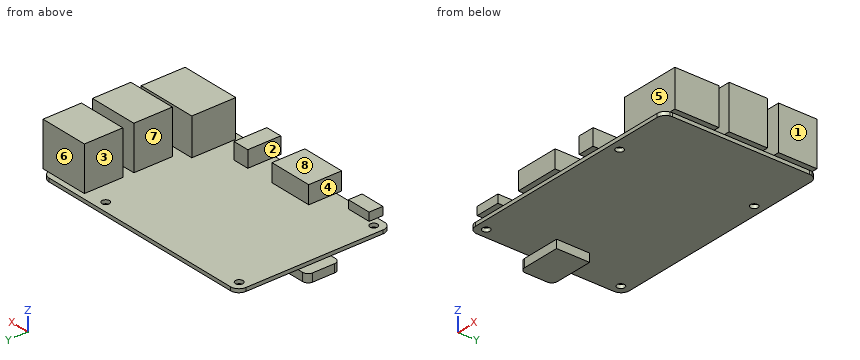
```python
from build123d import *

# Parameters (mm, degrees)
F0_R     = 1.375
F0_W     = 9
F0_H     = 3
F0_W_2   = 16
F0_H_2   = 10
F0_W_3   = 6
F0_H_3   = 14
F1_DEPTH = 1.3
F0_W_4   = 2
F2_DEPTH = 16
F3_DEPTH = 13.5
F0_H_4   = 2
F4_DEPTH = 6
F5_DEPTH = 6.5
F6_DEPTH = 3
F7_W     = 4
F7_H     = 12
F7_W_2   = 12
F8_DEPTH = 3
F9_R     = 2


# Not quite as in the source:
# - a feature names something its author has since deleted; it is built from what else it names


with BuildPart() as f1:
    # F0 (on Top) → F1 (new body)
    with BuildSketch(Plane.XY):
        with BuildLine():
            Line((-28.5, 0), (-3, 0))
            ThreePointArc((-3, 0), (-1.1628826929, 0.6282917549), (-0.0952624903, 2.25))
            Line((-0.0952624903, 2.25), (-20, 2.25))
            Line((-20, 2.25), (-20, 18.25))
            Line((-20, 18.25), (0, 18.25))
            Line((0, 18.25), (0, 22))
            Line((0, 22), (-16, 22))
            Line((-16, 22), (-16, 36))
            Line((-16, 36), (0, 36))
            Line((0, 36), (0, 40))
            Line((0, 40), (-16, 40))
            Line((-16, 40), (-16, 54))
            Line((-16, 54), (-0.1715728753, 54))
            ThreePointArc((-0.1715728753, 54), (-1.2679491924, 55.4494897428), (-3, 56))
            Line((-3, 56), (-82, 56))
            ThreePointArc((-82, 56), (-84.1213203436, 55.1213203436), (-85, 53))
            Line((-85, 53), (-85, 3))
            ThreePointArc((-85, 3), (-84.1213203436, 0.8786796564), (-82, 0))
            Line((-82, 0), (-78.9, 0))
            Line((-78.9, 0), (-78.9, 3))
            Line((-78.9, 3), (-69.9, 3))
            Line((-69.9, 3), (-69.9, 0))
            Line((-69.9, 0), (-61, 0))
            Line((-61, 0), (-61, 10))
            Line((-61, 10), (-45, 10))
            Line((-45, 10), (-45, 0))
            Line((-45, 0), (-34.5, 0))
            Line((-34.5, 0), (-34.5, 10))
            Line((-34.5, 10), (-28.5, 10))
            Line((-28.5, 10), (-28.5, 0))
        make_face()
        with Locations((-81.5, 3.5)):
            Circle(F0_R, mode=Mode.SUBTRACT)
        with Locations((-23.5, 3.5)):
            Circle(F0_R, mode=Mode.SUBTRACT)
        with Locations((-81.5, 52.5)):
            Circle(F0_R, mode=Mode.SUBTRACT)
        with Locations((-23.5, 52.5)):
            Circle(F0_R, mode=Mode.SUBTRACT)
        with Locations((-74.4, 1.5)):
            Rectangle(F0_W, F0_H)
        with Locations((-53, 5)):
            Rectangle(F0_W_2, F0_H_2)
        with Locations((-31.5, 5)):
            Rectangle(F0_W_3, F0_H_2)
        with BuildLine():
            Line((-20, 2.25), (-0.0952624903, 2.25))
            ThreePointArc((-0.0952624903, 2.25), (-0.0239109112, 2.6219871226), (0, 3))
            Line((0, 3), (0, 18.25))
            Line((0, 18.25), (-20, 18.25))
            Line((-20, 18.25), (-20, 2.25))
        make_face()
        with Locations((-8, 29)):
            Rectangle(F0_W_2, F0_H_3)
        with BuildLine():
            Line((-16, 40), (0, 40))
            Line((0, 40), (0, 53))
            ThreePointArc((0, 53), (-0.043204321, 53.5073059362), (-0.1715728753, 54))
            Line((-0.1715728753, 54), (-16, 54))
            Line((-16, 54), (-16, 40))
        make_face()
    extrude(amount=-F1_DEPTH)

    # F0 (on Top) → F2 (join)
    with BuildSketch(Plane.XY):
        with BuildLine():
            Line((-16, 40), (0, 40))
            Line((0, 40), (0, 53))
            ThreePointArc((0, 53), (-0.043204321, 53.5073059362), (-0.1715728753, 54))
            Line((-0.1715728753, 54), (-16, 54))
            Line((-16, 54), (-16, 40))
        make_face()
        with Locations((-8, 29)):
            Rectangle(F0_W_2, F0_H_3)
        with Locations((1, 29)):
            Rectangle(F0_W_4, F0_H_3)
        with BuildLine():
            Line((0, 53), (0, 40))
            Line((0, 40), (2, 40))
            Line((2, 40), (2, 54))
            Line((2, 54), (-0.1715728753, 54))
            ThreePointArc((-0.1715728753, 54), (-0.043204321, 53.5073059362), (0, 53))
        make_face()
    extrude(amount=F2_DEPTH)

    # F0 (on Top) → F3 (join)
    with BuildSketch(Plane.XY):
        with BuildLine():
            Line((-20, 2.25), (-0.0952624903, 2.25))
            ThreePointArc((-0.0952624903, 2.25), (-0.0239109112, 2.6219871226), (0, 3))
            Line((0, 3), (0, 18.25))
            Line((0, 18.25), (-20, 18.25))
            Line((-20, 18.25), (-20, 2.25))
        make_face()
        with BuildLine():
            ThreePointArc((0, 3), (-0.0239109112, 2.6219871226), (-0.0952624903, 2.25))
            Line((-0.0952624903, 2.25), (2, 2.25))
            Line((2, 2.25), (2, 18.25))
            Line((2, 18.25), (0, 18.25))
            Line((0, 18.25), (0, 3))
        make_face()
    extrude(amount=F3_DEPTH)

    # F0 (on Top) → F4 (join)
    with BuildSketch(Plane.XY):
        with Locations((-31.5, -1)):
            Rectangle(F0_W_3, F0_H_4)
        with Locations((-31.5, 5)):
            Rectangle(F0_W_3, F0_H_2)
    extrude(amount=F4_DEPTH)

    # F0 (on Top) → F5 (join)
    with BuildSketch(Plane.XY):
        with Locations((-53, 5)):
            Rectangle(F0_W_2, F0_H_2)
        with Locations((-53, -1)):
            Rectangle(F0_W_2, F0_H_4)
    extrude(amount=F5_DEPTH)

    # F0 (on Top) → F6 (join)
    with BuildSketch(Plane.XY):
        with Locations((-74.4, 1.5)):
            Rectangle(F0_W, F0_H)
        with Locations((-74.4, -1)):
            Rectangle(F0_W, F0_H_4)
    extrude(amount=F6_DEPTH)

    # F7 (on face) → F8 (join)
    with BuildSketch(Plane(origin=(0, 0, -1.3), x_dir=(1, 0, 0), z_dir=(0, 0, -1))):
        with Locations((-87, -28)):
            Rectangle(F7_W, F7_H)
        with Locations((-79, -28)):
            Rectangle(F7_W_2, F7_H)
    extrude(amount=F8_DEPTH)

    # F9
    f9_edges = [f1.edges().sort_by_distance(p)[0] for p in [
        (-89, 22, -2.8),
        (-89, 34, -2.8),
    ]]
    fillet(f9_edges, radius=F9_R)


solid = f1.part
```
The listing builds one solid part. Answer for the finished solid, in the listing's coordinates (mm). Face numbers are marked on the shaded views. A direction names the side the tool comes from. Coordinates: 2 decimals unless noted, no trailing zeros. Write each loop counter-clockwise with the first axis right and the second up, starting at its lowest first coordinate (ties: lowest second). Pieces come first, ordered by that corner, then holes. Notation, with made-up numbers: (1.25, -6) -> (57.25, -6) arc R8 cw to (57.25, 7) -> close; hole circle Ø2 at (51.25, -1.75). An arc over 180 degrees is marked (long way). Write each question's results on one line, items separated by ' | '. Start each with the question number.
1) A cutting plane is placed at D-D (x = -51.5). Determine the outline of the cut face in (y, z), then the cut area to 3 significant figures.
2) Flat-ended cylindrical pins translate along their axes: pin 1 Ø2.5 at (x, z) = (-72.5, 2) entering from +Y; pin 2 Ø12 at (x, y) = (-64, 4.5) entering from +Z; pin 3 Ø3 at (x, y) = (-23.5, 52.5) entering from -Z. Find the tip coordinate at first contact, or state that the pin passes through.
3) A cutting plane is placed at B-B (z = 8.75). Determine the outline of the cut face in (x, y), then the cut area to 3 significant figures.
4) A tool of negligible diameter and unlimited length cuts with its end or side. For the marked faces 5, 6, 7 and 8, from which of +Z, -Z, +X, -X, +Y, -Y can it reach the whole face along a straight path? Write none if from no direction.
5) A cutting plane is placed at A-A (x = -23.5). Determine the outline of the cut face in (y, z) (3 decimals), then the cut area to 4 significant figures.
6) For a pull along X with two mould halves and no side action, classify the marked faces 1, 2, 3 and 4 as +X half, -X half, draft (parallel to the pull), parting line (faces both ways), or undercut.
7) Straight lines are drawn through the part: probe 1 along X at (y, z) = (9, 5.5); probe 2 along Y at (x, z) = (-23.5, -0.75) (3 decimals); probe 3 along Y at (x, z) = (-34.5, -1). For each, find the intervals that lie inside material, in ascending order.
8) A cutting plane is placed at C-C (y = 9). Determine the outline of the cut face in (x, z).
Values follow:
1) outline: (-2, 0) -> (0, 0) -> (0, -1.3) -> (56, -1.3) -> (56, 0) -> (10, 0) -> (10, 6.5) -> (-2, 6.5) -> close | area: 151 mm²
2) pin 1: y = 3 | pin 2: z = 6.5 | pin 3: z = -1.3
3) outline: (-20, 2.25) -> (2, 2.25) -> (2, 18.25) -> (-20, 18.25) -> close; (-16, 22) -> (2, 22) -> (2, 36) -> (-16, 36) -> close; (-16, 40) -> (2, 40) -> (2, 54) -> (-16, 54) -> close | area: 856 mm²
4) face 5: +Z, +X, -Y | face 6: +Z, +X, -X, +Y | face 7: +Z, -X, +Y | face 8: +Z, -X, +Y, -Y
5) outline: (0, -1.3) -> (2.125, -1.3) -> (2.125, 0) -> (0, 0) -> close; (4.875, -1.3) -> (51.125, -1.3) -> (51.125, 0) -> (4.875, 0) -> close; (53.875, -1.3) -> (56, -1.3) -> (56, 0) -> (53.875, 0) -> close | area: 65.65 mm²
6) face 1: +X half | face 2: undercut | face 3: -X half | face 4: undercut
7) probe 1: -61 to -45, -34.5 to -28.5, -20 to 2 | probe 2: 0 to 2.125, 4.875 to 51.125, 53.875 to 56 | probe 3: 0 to 56
8) outline: (-85, -1.3) -> (0, -1.3) -> (0, 0) -> (2, 0) -> (2, 13.5) -> (-20, 13.5) -> (-20, 0) -> (-28.5, 0) -> (-28.5, 6) -> (-34.5, 6) -> (-34.5, 0) -> (-45, 0) -> (-45, 6.5) -> (-61, 6.5) -> (-61, 0) -> (-85, 0) -> close
